```python
from build123d import *

# Parameters (mm, degrees)
EXTRUDE_1_DEPTH    = 30
HOLE_WIZARD_M8_1_D = 6.8
EXTRUDE_2_DEPTH    = 12


with BuildPart() as part:
    # 草图1 → 凸台-拉伸1 (new body, symmetric)
    with BuildSketch(Plane.XY):
        with BuildLine():
            Line((-21, 0), (21, 0))
            Line((21, 0), (22, 1))
            Line((22, 1), (35, 1))
            Line((35, 1), (35, -9))
            Line((35, -9), (32.639225352, -9))
            ThreePointArc((32.639225352, -9), (30.19452262, -9.638414445), (28.374113304, -11.390628579))
            ThreePointArc((28.374113304, -11.390628579), (24.899602423, -19.616168903), (24, -28.5))
            Line((24, -28.5), (11.5, -28.5))
            Line((11.5, -28.5), (11.5, -13))
            Line((11.5, -13), (-11.5, -13))
            Line((-11.5, -13), (-11.5, -28.5))
            Line((-11.5, -28.5), (-24, -28.5))
            ThreePointArc((-24, -28.5), (-24.899602423, -19.616168903), (-28.374113304, -11.390628579))
            ThreePointArc((-28.374113304, -11.390628579), (-30.19452262, -9.638414445), (-32.639225352, -9))
            Line((-32.639225352, -9), (-35, -9))
            Line((-35, -9), (-35, 1))
            Line((-35, 1), (-22, 1))
            Line((-22, 1), (-21, 0))
        make_face()
    extrude(amount=EXTRUDE_1_DEPTH, both=True)

    # M8 螺纹孔1 (through all)
    with Locations(Plane(origin=(0, 1, 0), x_dir=(1, 0, 0), z_dir=(0, 1, 0))):
        with Locations((-28.5, 22.5), (28.5, 22.5), (28.5, -22.5), (-28.5, -22.5)):
            Hole(HOLE_WIZARD_M8_1_D / 2)

    # 草图4 → 凸台-拉伸2 (add)
    with BuildSketch(Plane.XY.offset(30)):
        Polygon((-11.5, -28.5), (-11.5, -13), (11.5, -13), (11.5, -28.5), (24, -28.5), (24, -1.5), (-24, -1.5), (-24, -28.5), align=None)
    extrude_2 = extrude(amount=EXTRUDE_2_DEPTH)

    # 镜向1: 凸台-拉伸2 across plane
    add(extrude_2.mirror(Plane.XY))


solid = part.part
```
Input: part model. Units: mm. Frame: model coordinates. A direction names the side the tool comes from. Coordinates: 2 decimals unless noted, no trailing zeros. Write each loop counter-clockwise with the first axis right and the second up, starting at its lowest first coordinate (ties: lowest second). Pieces come first, ordered by that corner, then holes. Notation, with made-up numbers: M 79.5,-0.75 L 84.5,-0.75 A19 ccw 84.5,31.25 Z; hole C 88,49.5 d10. An arc over 180 degrees is marked long. Use one line per item in the form item = value.
Q1. Section A-A (z = 36.5). Return loops of the section in (x, y), plus the area to 4 significant figures.
Answer below:
outline = M -24,-28.5 L -11.5,-28.5 L -11.5,-13 L 11.5,-13 L 11.5,-28.5 L 24,-28.5 L 24,-1.5 L -24,-1.5 Z
area = 939.5 mm²
Q2. Material intervals for probe 1 along Z at (x, y) = (-28.5, -5.25); probe 2 along X at (y, z) = (-26, 38); probe 3 along Y at (x, z) = (-15, -10.5), sorted ascending. Write a range as from..to.
Answer below:
probe_1 = -30..-25.9, -19.1..19.1, 25.9..30
probe_2 = -24..-11.5, 11.5..24
probe_3 = -28.5..0
Q3. Section C-C (y = -6.5). Return loops of the section in (x, z), plus the area to 3 significant figures.
Answer below:
outline = M -35,-30 L -24,-30 L -24,-42 L 24,-42 L 24,-30 L 35,-30 L 35,30 L 24,30 L 24,42 L -24,42 L -24,30 L -35,30 Z; hole C -28.5,-22.5 d6.8; hole C -28.5,22.5 d6.8; hole C 28.5,-22.5 d6.8; hole C 28.5,22.5 d6.8
area = 5,210 mm²
Q4. Set-up query: faces 5 (the face through (-34, -9, 0)), 6 (the face through (11.5, -21, 1)), 7 (the face through (34, -9, 0)), 8 (the face through (0, -1.5, 36)), 9 (the face through (-24, -15, 36)). Return all of +Z, -Z, +X, -X, +Y, -Y with unobstructed straight access to the full face (end or side cutting, diameter ignored); none if empty.
Answer below:
face_5 = +Z, -Z, -X, -Y
face_6 = +Z, -Z, -Y
face_7 = +Z, -Z, +X, -Y
face_8 = +Z, +X, -X, +Y
face_9 = +Z, -X, +Y, -Y
Q5. First-contact query: pin 1 (6 mm diameter, centred on x = 6, z = -34, fed in from +Y); pin 2 (6 mm diameter, centred on y = -19, z = -35.5, fed in from -X); pin 3 (8 mm diameter, centred on y = -22, z = -13.5, fed in from -X). Flat tips, straight axial feed; report the tip coordinate or a pass-through.
Answer below:
pin_1 = -1.5
pin_2 = -24
pin_3 = -25.36
Q6. Section D-D (z = -22.5). Return loops of the section in (x, y).
Answer below:
outline = M -35,-9 L -32.64,-9 A5 cw -31.9,-9.05 L -31.9,1 L -35,1 Z; M -25.1,-18.87 A30 cw -24,-28.5 L -11.5,-28.5 L -11.5,-13 L 11.5,-13 L 11.5,-28.5 L 24,-28.5 A30 cw 25.1,-18.87 L 25.1,1 L 22,1 L 21,0 L -21,0 L -22,1 L -25.1,1 Z; M 31.9,-9.05 A5 cw 32.64,-9 L 35,-9 L 35,1 L 31.9,1 Z
Q7. Section B-B (x = 19). Return loops of the section in (y, z), plus the area to 3 significant figures.
Answer below:
outline = M -28.5,-42 L -1.5,-42 L -1.5,-30 L 0,-30 L 0,30 L -1.5,30 L -1.5,42 L -28.5,42 Z
area = 2,360 mm²
Q8. Draft query along Z for faces 1 (the face through (0, -12, -42)), 2 (the face through (24, -15, -36)), 3 (the face through (-25.1, -6.9, 22.4)), 4 (the face through (25.36, -6.87, 23.8)). Return one class per face: released by +Z, released by -Z, zero draft, split by the parting line, or undercut.
Answer below:
face_1 = released by -Z
face_2 = zero draft
face_3 = undercut
face_4 = undercut
